Input: part model. Units: mm. Frame: model coordinates. A direction names the side the tool comes from. Round coordinates to 2 decimals unless told otherwise and drop trailing zeros. Order: outer loops, then holes, each group sorted by start corner. A loop starts at its lowest first (then second) coordinate and runs counter-clockwise, first axis right, second up. Notation, with made-up numbers: (-2.75, 19.5) - (19.25, 19.5) arc R29 cw to (19.25, 46.5) - close; hole circle Ø5 at (-33, 45.5). An arc over 180 degrees is marked (long way). One line per item, written item: value. Start each with the question number.
from build123d import *

# Parameters (mm, degrees)
F1_DEPTH = 60
F2_W     = 70
F2_H     = 15
F3_DEPTH = 50
F4_R     = 15
F5_R     = 15
F6_DEPTH = 67.5


with BuildPart() as f1:
    # F0 (on Front) → F1 (new body)
    with BuildSketch(Plane.XZ):
        with BuildLine():
            Line((-8.039089, 59.247605), (-48.039089, 59.247605))
            Line((-48.039089, 59.247605), (-48.039089, 49.157878))
            ThreePointArc((-48.039089, 49.157878), (-31.879825, 34.202742), (-48.039089, 19.247605))
            Line((-48.039089, 19.247605), (-48.039089, -60.752395))
            Line((-48.039089, -60.752395), (-8.039089, -60.752395))
            Line((-8.039089, -60.752395), (-8.039089, -20.752395))
            Line((-8.039089, -20.752395), (11.960911, -20.752395))
            Line((11.960911, -20.752395), (11.960911, -60.752395))
            Line((11.960911, -60.752395), (51.960911, -60.752395))
            Line((51.960911, -60.752395), (51.960911, 19.247605))
            ThreePointArc((51.960911, 19.247605), (35.801647, 34.202742), (51.960911, 49.157878))
            Line((51.960911, 49.157878), (51.960911, 59.247605))
            Line((51.960911, 59.247605), (11.960911, 59.247605))
            Line((11.960911, 59.247605), (11.960911, 19.247605))
            Line((11.960911, 19.247605), (-8.039089, 19.247605))
            Line((-8.039089, 19.247605), (-8.039089, 59.247605))
        make_face()
    extrude(amount=F1_DEPTH)

    # F2 (on face) → F3 (cut)
    with BuildSketch(Plane.XZ.offset(60)):
        with Locations((1.960911, -0.752395)):
            Rectangle(F2_W, F2_H)
    extrude(amount=-F3_DEPTH, mode=Mode.SUBTRACT)

    # F4 (on face) + F5 (on face) → F6 (cut)
    with BuildSketch(Plane(origin=(0, 0, -60.752395), x_dir=(1, 0, 0), z_dir=(0, 0, -1))):
        with Locations((-28.039089, 20)):
            Circle(F4_R)
    with BuildSketch(Plane(origin=(0, 0, -60.752395), x_dir=(1, 0, 0), z_dir=(0, 0, -1))):
        with Locations((31.960911, 20)):
            Circle(F5_R)
    extrude(amount=-F6_DEPTH, mode=Mode.SUBTRACT)


solid = f1.part
Item 1: Line query: L1, parallel to X at y = -20, z = -24; L2, parallel to X at y = -20, z = -8.5; L3, parallel to Z at x = 18, y = -27. Output: solid intervals per line, ascending.
Item 2: Section query C-C on y = -43. Return loops of the section in (x, z).
Item 3: Section query A-A on y = -20. Return loops of the section in (x, z), and give its area (3 significant figures).
Item 4: Section query B-B on z = -45.5. Return loops of the section in (x, y).
Item 5: Pull-direction query (Z, two-part tool) for faces 1 (the face through (1, -41, -8.252)), 2 (the face through (2, -30, 19.248)), 3 (the face through (-8.039, -30, -41)); classes: released by +Z, released by -Z, zero draft, split by the parting line, or undercut.
Item 6: Reachability of faces 4 (the face through (-33.039, -47, -1)), 5 (the face through (-39.94, -10.87, -27.47)), 6 (the face through (11.961, -30, 40)), 7 (the face through (11.961, -30, -40)) from +Z, -Z, +X, -X, +Y, -Y: full face, straight path, thin tool, end or side. Return the list, or none.
Item 7: First-contact query: pin 1 Ø1 at (x, z) = (30.5, 40.5) entering from +Y; pin 2 Ø4.5 at (x, z) = (-2, -1.5) entering from -Y; pin 3 Ø5 at (x, y) = (-35.5, -14.5) entering from -Z; pin 4 Ø12 at (y, z) = (-27.5, 41.5) entering from -X. Flat tips, straight axial feed; report the tip coordinate or a pass-through.
Item 8: Section query D-D on z = -4. Return loops of the section in (x, y).
Geometry results:
1. L1: x = -48.04 to -43.04, -13.04 to -8.04, 11.96 to 16.96, 46.96 to 51.96
1. L2: x = -48.04 to -43.04, -13.04 to 16.96, 46.96 to 51.96
1. L3: z = -60.75 to -8.25, 6.75 to 59.25
2. outline: (-48.04, -60.75) - (-8.04, -60.75) - (-8.04, -20.75) - (11.96, -20.75) - (11.96, -60.75) - (51.96, -60.75) - (51.96, 19.25) arc R15 cw (long way) to (51.96, 49.16) - (51.96, 59.25) - (11.96, 59.25) - (11.96, 19.25) - (-8.04, 19.25) - (-8.04, 59.25) - (-48.04, 59.25) - (-48.04, 49.16) arc R15 cw (long way) to (-48.04, 19.25) - close; hole (-33.04, -8.25) - (36.96, -8.25) - (36.96, 6.75) - (-33.04, 6.75) - close
3. outline: (-48.04, -60.75) - (-43.04, -60.75) - (-43.04, 6.75) - (46.96, 6.75) - (46.96, -60.75) - (51.96, -60.75) - (51.96, 19.25) arc R15 cw (long way) to (51.96, 49.16) - (51.96, 59.25) - (11.96, 59.25) - (11.96, 19.25) - (-8.04, 19.25) - (-8.04, 59.25) - (-48.04, 59.25) - (-48.04, 49.16) arc R15 cw (long way) to (-48.04, 19.25) - close; (-13.04, -60.75) - (-8.04, -60.75) - (-8.04, -20.75) - (11.96, -20.75) - (11.96, -60.75) - (16.96, -60.75) - (16.96, -8.25) - (-13.04, -8.25) - close
3. area: 5,120 mm^2
4. outline: (-48.04, -60) - (-8.04, -60) - (-8.04, 0) - (-48.04, 0) - close; (11.96, -60) - (51.96, -60) - (51.96, 0) - (11.96, 0) - close; hole circle Ø30 at (-28.04, -20); hole circle Ø30 at (31.96, -20)
5. face 1: undercut
5. face 2: released by +Z
5. face 3: zero draft
6. face 4: -Y
6. face 5: -Z
6. face 6: +Z, +Y, -Y
6. face 7: -Z, +Y, -Y
7. pin 1: stops at y = 0
7. pin 2: stops at y = -10
7. pin 3: stops at z = 6.75
7. pin 4: stops at x = -39.94
8. outline: (-48.04, -60) - (-33.04, -60) - (-33.04, -34.14) arc R15 cw (long way) to (-16.86, -10) - (20.78, -10) arc R15 cw (long way) to (36.96, -34.14) - (36.96, -60) - (51.96, -60) - (51.96, 0) - (-48.04, 0) - close
